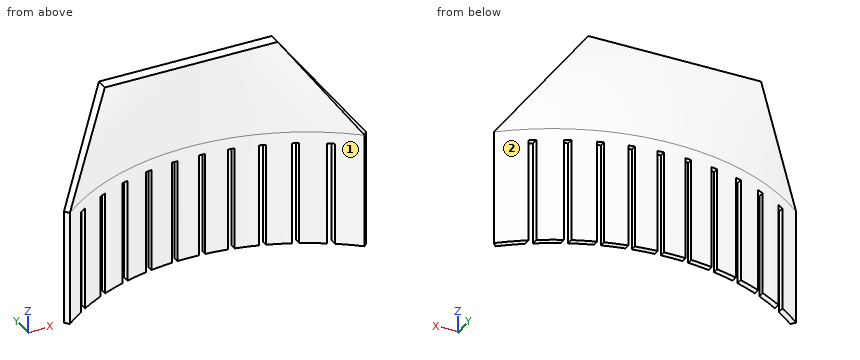
from build123d import *

# Parameters (mm, degrees)
F1_DEPTH = 20
F2_W     = 1.029727
F2_H     = 13.097165
F3_DEPTH = 18
F5_W     = 30
F5_H     = 2


with BuildPart() as f1:
    # F0 (on Top) → F1 (new body)
    with BuildSketch(Plane.XY):
        with BuildLine():
            ThreePointArc((-25.586572, 0), (0, 9.300989), (25.586572, 0))
            Line((25.586572, 0), (26.228737, 0.766566))
            ThreePointArc((26.228737, 0.766566), (0, 10.300989), (-26.228737, 0.766566))
            Line((-26.228737, 0.766566), (-25.586572, 0))
        make_face()
    extrude(amount=F1_DEPTH)

    # F2 (on Top) → F3 (cut)
    with BuildSketch(Plane.XY):
        with Locations((-21.875679, 6.548582)):
            Rectangle(F2_W, F2_H)
        with Locations((-17.075679, 6.548582)):
            Rectangle(F2_W, F2_H)
        with Locations((-12.275679, 6.548582)):
            Rectangle(F2_W, F2_H)
        with Locations((-7.47568, 6.548582)):
            Rectangle(F2_W, F2_H)
        with Locations((-2.67568, 6.548582)):
            Rectangle(F2_W, F2_H)
        with Locations((2.12432, 6.548582)):
            Rectangle(F2_W, F2_H)
        with Locations((6.924321, 6.548582)):
            Rectangle(F2_W, F2_H)
        with Locations((11.72432, 6.548582)):
            Rectangle(F2_W, F2_H)
        with Locations((16.52432, 6.548582)):
            Rectangle(F2_W, F2_H)
        with Locations((21.32432, 6.548582)):
            Rectangle(F2_W, F2_H)
    extrude(amount=F3_DEPTH, mode=Mode.SUBTRACT)

    # F1_face (on face) → F6 section 0
    with BuildSketch(Plane(origin=(0, 6.611875, 20), x_dir=(1, 0, 0), z_dir=(0, 0, 1))):
        with BuildLine():
            Line((25.586572, -6.611875), (26.228737, -5.845309))
            ThreePointArc((26.228737, -5.845309), (0, 3.689114), (-26.228737, -5.845309))
            Line((-26.228737, -5.845309), (-25.586572, -6.611875))
            ThreePointArc((-25.586572, -6.611875), (0, 2.689114), (25.586572, -6.611875))
        make_face()
    # F5 (on offset) → F6 section 1
    with BuildSketch(Plane.XY.offset(35)):
        with Locations((0, 9.8)):
            Rectangle(F5_W, F5_H)
    loft()


solid = f1.part
Check sheet for the modelled part. Datum: model origin and axes. Units: mm. Face numbers are marked on the shaded views. A direction names the side the tool comes from. Round coordinates to 2 decimals unless told otherwise and drop trailing zeros. One line per item, written item: value.
(1) Depth check by flat-ended pin: pin 1 Ø6 at (x, z) = (8.5, 22.5) entering from +Y; pin 2 Ø0.6 at (y, z) = (4, 13.5) entering from -X; pin 3 Ø0.8 at (x, y) = (-17, 5.5) entering from -Z; pin 4 Ø3 at (x, y) = (-2, 7) entering from -Z. Enter the tip coordinate at first touch or a pass-through.
Computed values:
pin 1: stops at y = 10.03
pin 2: stops at x = -21.36
pin 3: stops at z = 18
pin 4: passes through
(2) Thickness scan on line 1 (X direction, y = 3.75, z = 15.5); line 2 (Y direction, x = 0.5, z = 4); line 3 (X direction, y = 1, z = 21). Record the ranges inside material, lowest first.
Computed values:
line 1: x = -21.36 to -20.29, 20.29 to 20.81, 21.84 to 22.19
line 2: y = 9.3 to 10.3
line 3: x = -25.17 to -24.35, 24.35 to 25.17
(3) Sectioned sample at A-A, the plane z = 4. Count the separate pieces of the cut face and the enclosed holes in it, then the cut area to 3 significant figures.
Computed values:
separate pieces: 11
enclosed holes: 0
area: 45.2 mm^2
(4) Access from +Z, -Z, +X, -X, +Y, -Y to the whole of each face (thin tool, end or side, straight path). Record for the marked faces 1 and 2.
Computed values:
face 1: -Z, -Y
face 2: -Z, +Y
